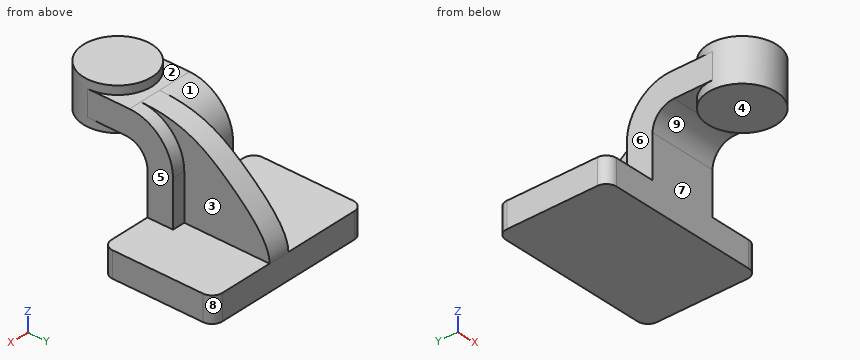
```python
from build123d import *

# Parameters (mm, degrees)
F1_DEPTH = 9.525
F3_DEPTH = 25.4
F5_R     = 25.4
F6_DEPTH = 15.875
F8_DEPTH = 15.875


with BuildPart() as f1:
    # F0 (on Top) → F1 (new body, symmetric)
    with BuildSketch(Plane.XY):
        with BuildLine():
            ThreePointArc((63.5, 33.655), (61.2681536726, 39.0431536726), (55.88, 41.275))
            Line((55.88, 41.275), (-55.88, 41.275))
            ThreePointArc((-55.88, 41.275), (-61.2681536726, 39.0431536726), (-63.5, 33.655))
            Line((-63.5, 33.655), (-63.5, -33.655))
            ThreePointArc((-63.5, -33.655), (-61.2681536726, -39.0431536726), (-55.88, -41.275))
            Line((-55.88, -41.275), (55.88, -41.275))
            ThreePointArc((55.88, -41.275), (61.2681536726, -39.0431536726), (63.5, -33.655))
            Line((63.5, -33.655), (63.5, 33.655))
        make_face()
    extrude(amount=F1_DEPTH, both=True)

    # F2 (on Right) → F3 (join, symmetric)
    with BuildSketch(Plane.YZ):
        with BuildLine():
            Line((-41.275, 9.525), (-22.225, 9.525))
            Line((-22.225, 9.525), (-22.225, 43.815))
            ThreePointArc((-22.225, 43.815), (-31.7103468913, 66.7146531087), (-54.61, 76.2))
            Line((-54.61, 76.2), (-85.725, 76.2))
            Line((-85.725, 76.2), (-85.725, 57.15))
            Line((-85.725, 57.15), (-57.15, 57.15))
            ThreePointArc((-57.15, 57.15), (-45.9246798487, 52.5003201513), (-41.275, 41.275))
            Line((-41.275, 41.275), (-41.275, 9.525))
        make_face()
    extrude(amount=F3_DEPTH, both=True)

    # F5 (on mid) → F6 (join, symmetric)
    with BuildSketch(Plane.XY.offset(66.675)):
        with Locations((0, -85.725)):
            Circle(F5_R)
    extrude(amount=F6_DEPTH, both=True)

    # F7 (on Right) → F8 (join)
    with BuildSketch(Plane.YZ):
        with BuildLine():
            ThreePointArc((-54.61, 76.2), (-31.7103468913, 66.7146531087), (-22.225, 43.815))
            Line((-22.225, 43.815), (-22.225, 9.525))
            Line((-22.225, 9.525), (41.275, 9.525))
            add(Edge.make_bspline(
                [(-54.61, 76.2), (-22.4902851436, 76.2), (7.474900406, 55.7835251702), (41.275, 23.4287642155), (41.275, 9.525)],
                knots=[0, 0, 0, 0, 0.4371907779, 0.8096505074, 0.8096505074, 0.8096505074, 0.8096505074], degree=3))
        make_face()
    extrude(amount=F8_DEPTH)


solid = f1.part
```
For this review, take the finished solid that the model builds, in its own axes (mm). Face numbers are marked on the shaded views. A direction names the side the tool comes from. Round coordinates to 2 decimals unless told otherwise and drop trailing zeros. Order: outer loops, then holes, each group sorted by start corner. A loop starts at its lowest first (then second) coordinate and runs counter-clockwise, first axis right, second up.
Q1. Mouldability with a two-part tool opening along Y and no side actions: class the marked faces 6, 7, 8 and 9 as pulls with the +Y half, pulls with the -Y half, needs draft (parallel to the pull), parting line crosses it, or undercut.
Findings below:
face 6: needs draft
face 7: pulls with the -Y half
face 8: pulls with the +Y half
face 9: undercut
Q2. We need section B-B, the plane z = 7.5. Give the boundary of the cut face in (x, y) (3 decimals).
Findings below:
outline: (-63.5, -33.655) arc R7.62 ccw to (-55.88, -41.275) - (55.88, -41.275) arc R7.62 ccw to (63.5, -33.655) - (63.5, 33.655) arc R7.62 ccw to (55.88, 41.275) - (-55.88, 41.275) arc R7.62 ccw to (-63.5, 33.655) - close
Q3. Insertion check: P1, Ø24, axis at x = 42, y = 6.5, coming from the +Z side (3 decimals); P2, Ø12, axis at x = 21, y = -70, coming from the -Z side; P3, Ø10, axis at y = -33.5, z = 19, coming from the -X side. Each pin has a flat end and moves straight along its axis. Give the tip position at first contact, or say it passes through.
Findings below:
P1: stops at z = 9.525
P2: stops at z = 50.8
P3: stops at x = -25.4
Q4. We need section A-A, the plane x = -3. Give the boundary of the cut face in (y, z) (3 decimals), plus the area to 3 significant figures.
Findings below:
outline: (-110.947, 50.8) - (-60.503, 50.8) - (-60.503, 57.15) - (-57.15, 57.15) arc R15.875 cw to (-41.275, 41.275) - (-41.275, -9.525) - (41.275, -9.525) - (41.275, 9.525) - (-22.225, 9.525) - (-22.225, 43.815) arc R32.385 ccw to (-54.61, 76.2) - (-60.503, 76.2) - (-60.503, 82.55) - (-110.947, 82.55) - close
area: 4,640 mm2
Q5. We need section C-C, the plane x = 19. Give the boundary of the cut face in (y, z) (3 decimals).
Findings below:
outline: (-102.582, 50.8) - (-68.868, 50.8) - (-68.868, 57.15) - (-57.15, 57.15) arc R15.875 cw to (-41.275, 41.275) - (-41.275, -9.525) - (41.275, -9.525) - (41.275, 9.525) - (-22.225, 9.525) - (-22.225, 43.815) arc R32.385 ccw to (-54.61, 76.2) - (-68.868, 76.2) - (-68.868, 82.55) - (-102.582, 82.55) - close
Q6. We need section D-D, the plane x = 45.5. Give the boundary of the cut face in (y, z) (3 decimals), plus the area to 3 significant figures.
Findings below:
outline: (-41.275, -9.525) - (41.275, -9.525) - (41.275, 9.525) - (-41.275, 9.525) - close
area: 1,570 mm2
Q7. Wall thickness on line 1 (X direction, y = 12, z = 10) (3 decimals); line 2 (Z direction, x = -10.5, y = -79); line 3 (Y direction, x = 53, z = 2) (3 decimals): over which ranges is each line inside the solid? List them lowest first.
Findings below:
line 1: x = 0 to 15.875
line 2: z = 50.8 to 82.55
line 3: y = -41.275 to 41.275
Q8. Machinability: for the marked faces 1, 2, 3, 4 and 5, which of the approach directions +Z, -Z, +X, -X, +Y, -Y give a long, thin tool a straight path to every point of the face, cutting with its end or side? Answer none if there is none.
Findings below:
face 1: +Z, -X, +Y
face 2: +Z, +Y
face 3: +Z, +X, +Y
face 4: -Z, +X, -X, -Y
face 5: +Z, +X, +Y, -Y
